Answer from the drawing. Dimensions are ordinates in mm from the lowest x, y and z of the part. A direction names the side the tool comes from. Coordinates: 2 decimals unless noted, no trailing zeros. Write each loop counter-clockwise with the first axis right and the second up, starting at its lowest first coordinate (ties: lowest second). Pieces come first, ordered by that corner, then holes. Notation, with made-up numbers: (17.25, 35) -> (46.25, 35) arc R14 ccw to (46.25, 53) -> close; hole circle Ø1 at (-34, 75.25). An arc over 180 degrees is marked (long way). Use CSV: the item, a comma, the result in double quotes.
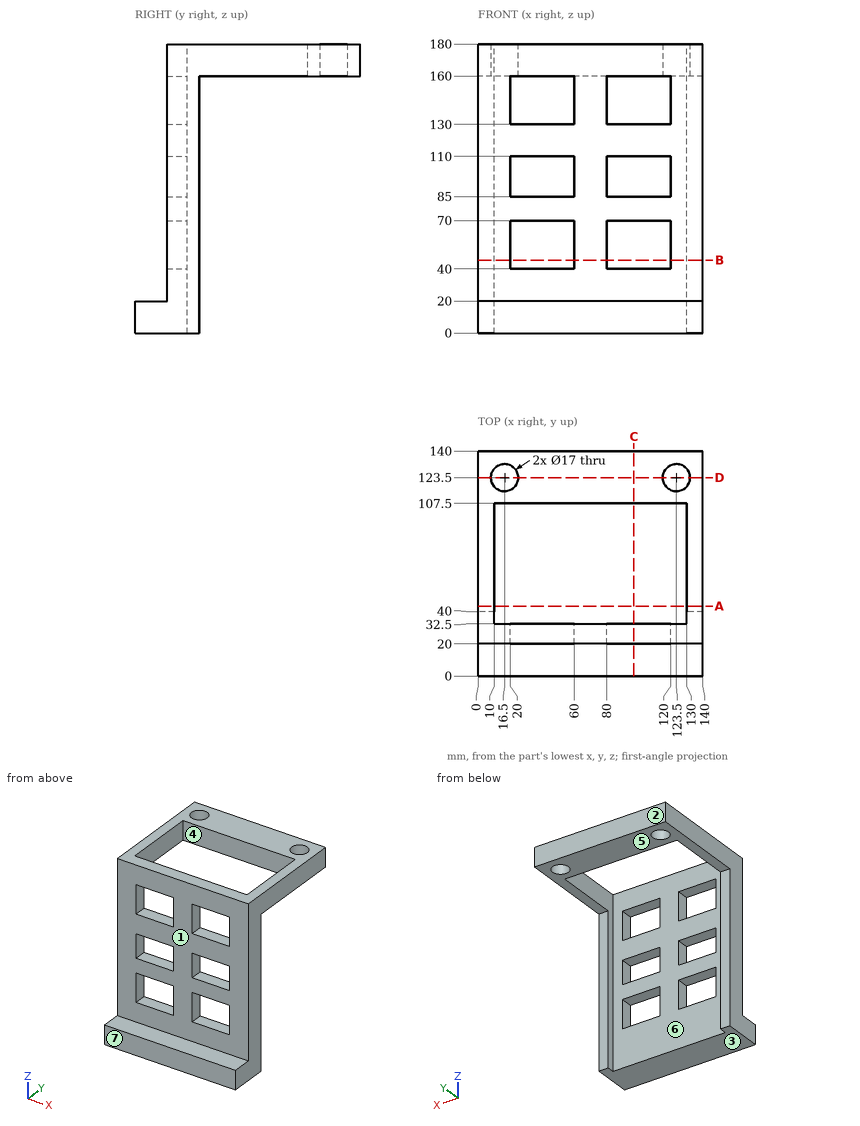
1. Find the intervals of material crossed by line 1 along X through (y, z) = (123, 165); line 2 along Y through (x, z) = (16.5, 167.5); line 3 along X through (y, z) = (31, 54), in increasing order.
Solutions:
line 1,"x = 0 to 8.01, 24.99 to 115.01, 131.99 to 140"
line 2,"y = 20 to 32.5, 107.5 to 115, 132 to 140"
line 3,"x = 0 to 20, 60 to 80, 120 to 140"
2. A cutting plane is placed at C-C (x = 97). Give the vertices of the cut face in (y, z), and give its area (3 significant figures).
Solutions:
outline,"(0, 0) -> (32.5, 0) -> (32.5, 40) -> (20, 40) -> (20, 20) -> (0, 20) -> close; (20, 70) -> (32.5, 70) -> (32.5, 85) -> (20, 85) -> close; (20, 110) -> (32.5, 110) -> (32.5, 130) -> (20, 130) -> close; (20, 160) -> (32.5, 160) -> (32.5, 180) -> (20, 180) -> close; (107.5, 160) -> (140, 160) -> (140, 180) -> (107.5, 180) -> close"
area,"2,240 mm^2"
3. A cutting plane is placed at B-B (z = 45.5). Give the vertices of the cut face in (x, y), and give its area (3 significant figures).
Solutions:
outline,"(0, 20) -> (20, 20) -> (20, 32.5) -> (10, 32.5) -> (10, 40) -> (0, 40) -> close; (60, 20) -> (80, 20) -> (80, 32.5) -> (60, 32.5) -> close; (120, 20) -> (140, 20) -> (140, 40) -> (130, 40) -> (130, 32.5) -> (120, 32.5) -> close"
area,"900 mm^2"
4. A tool of negligible diameter and unlimited length cuts with its end or side. For the marked faces 5, 6 and 7, from which of +Z, -Z, +X, -X, +Y, -Y can it reach the whole face along a straight path? Write none if from no direction.
Solutions:
face 5,"-Z, +X, -X, +Y"
face 6,"+Z, -Z"
face 7,"+Z, -Z, +X, -X, -Y"
5. For a pull along Y with two mould halves and no side action, classify the marked faces 1, 2, 3 and 4 as pulls with the +Y half, pulls with the -Y half, needs draft (parallel to the pull), parting line crosses it, or undercut.
Solutions:
face 1,"pulls with the -Y half"
face 2,"pulls with the +Y half"
face 3,"needs draft"
face 4,"undercut"
6. A cutting plane is placed at A-A (y = 43.5). Give the vertices of the cut face in (x, z).
Solutions:
outline,"(0, 160) -> (10, 160) -> (10, 180) -> (0, 180) -> close; (130, 160) -> (140, 160) -> (140, 180) -> (130, 180) -> close"
7. A cutting plane is placed at D-D (y = 123.5). Give the vertices of the cut face in (x, z).
Solutions:
outline,"(0, 160) -> (8, 160) -> (8, 180) -> (0, 180) -> close; (25, 160) -> (115, 160) -> (115, 180) -> (25, 180) -> close; (132, 160) -> (140, 160) -> (140, 180) -> (132, 180) -> close"
8. Each of these flat-tipped pins is pushed along its axis until it touches: pin 1 Ø12 at (x, z) = (40, 112) entering from -Y; pin 2 Ø12 at (x, y) = (50.5, 121) entering from -Z. Where does it stop, or does it pass through?
Solutions:
pin 1,"stops at y = 20"
pin 2,"stops at z = 160"
